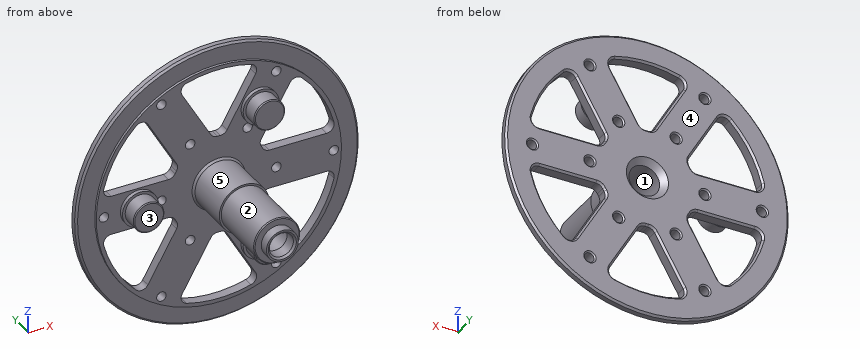
from build123d import *

# Parameters (mm, degrees)
CHAMFER1_SIZE                   = 0.5
CHAMFER2_SIZE                   = 0.25
CIRPATTERN1_COUNT               = 3
CHAMFER2_OF_CIRPATTERN1_SIZE    = 0.25
CHAMFER3_SIZE                   = 0.25
CHAMFER4_SIZE                   = 0.5
M3X0_5_TAPPED_HOLE1_D           = 2.5
M3X0_5_TAPPED_HOLE1_CSINK_D     = 3.2
M3X0_5_TAPPED_HOLE1_CSINK_ANGLE = 90
M3X0_5_TAPPED_HOLE2_D           = 2.5
M3X0_5_TAPPED_HOLE2_CSINK_D     = 3.2
M3X0_5_TAPPED_HOLE2_CSINK_ANGLE = 90
CIRPATTERN2_COUNT               = 6
CUT_EXTRUDE1_DEPTH              = 57.419943282
FILLET1_R                       = 2
CHAMFER5_SIZE                   = 0.5
CIRPATTERN3_COUNT               = 6
FILLET1_OF_CIRPATTERN3_R        = 2
CHAMFER5_OF_CIRPATTERN3_SIZE    = 0.5


with BuildPart() as part:
    # Sketch1 → Revolve1 (revolve)
    with BuildSketch(Plane.XY, mode=Mode.PRIVATE) as revolve1_sk:
        Polygon((-3.15, -8.7), (-4, -8.7), (-4, 19.6), (-5.5, 21.1), (-37, 21.1), (-37, 18.8), (-32, 18.8), (-32, 18.1), (-6.5, 18.1), (-6.5, 6), (-6, 6), (-6, 5.15), (-6, -6), (-6, -7.1), (-6, -9.7), (-4.15, -9.7), (-4.15, -12.2), (-3.15, -12.2), align=None)
    revolve(revolve1_sk.sketch.rotate(Axis((0, 0, 0), (0, -1, 0)), 270), axis=Axis((0, 0, 0), (0, -1, 0)))

    # Chamfer1
    chamfer1_edges = [part.edges().sort_by_distance(p)[0] for p in [
        (0, -12.2, -3.15),
    ]]
    chamfer(chamfer1_edges, length=CHAMFER1_SIZE)

    # Sketch2 → Planet bearing axis (revolve)
    with BuildSketch(Plane.XY):
        Polygon((-21, 18.1), (-25.7, 18.1), (-25.7, 17.1), (-25, 17.1), (-25, 13), (-21, 13), align=None)
    planet_bearing_axis = revolve(axis=Axis((-21, 33.164090746, 0), (0, -1, 0)))

    # Chamfer2
    chamfer2_edges = [part.edges().sort_by_distance(p)[0] for p in [
        (-17, 13, 0),
    ]]
    chamfer(chamfer2_edges, length=CHAMFER2_SIZE)

    # CirPattern1: Planet bearing axis ×3 about axis
    cirpattern1_axis = Axis((0, 0, 0), (0, 1, 0))
    for i in range(1, CIRPATTERN1_COUNT):
        add(planet_bearing_axis.rotate(cirpattern1_axis, i * 360 / CIRPATTERN1_COUNT))

    # Chamfer2 of CirPattern1
    chamfer2_of_cirpattern1_edges = [part.edges().sort_by_distance(p)[0] for p in [
        (8.5, 13, 14.722431864),
        (8.5, 13, -14.722431864),
    ]]
    chamfer(chamfer2_of_cirpattern1_edges, length=CHAMFER2_OF_CIRPATTERN1_SIZE)

    # Chamfer3
    chamfer3_edges = [part.edges().sort_by_distance(p)[0] for p in [
        (0, -9.7, -6),
    ]]
    chamfer(chamfer3_edges, length=CHAMFER3_SIZE)

    # Chamfer4
    chamfer4_edges = [part.edges().sort_by_distance(p)[0] for p in [
        (0, 18.1, -6.5),
        (0, 18.8, -37),
        (0, 21.1, -37),
    ]]
    chamfer(chamfer4_edges, length=CHAMFER4_SIZE)

    # M3x0.5 Tapped Hole1 (through all)
    with Locations(Plane(origin=(0, 21.1, 0), x_dir=(1, 0, 0), z_dir=(0, 1, 0))):
        with Locations((-30, 0)):
            m3x0_5_tapped_hole1 = CounterSinkHole(M3X0_5_TAPPED_HOLE1_D / 2, M3X0_5_TAPPED_HOLE1_CSINK_D / 2, counter_sink_angle=M3X0_5_TAPPED_HOLE1_CSINK_ANGLE)

    # M3x0.5 Tapped Hole2 (through all)
    with Locations(Plane(origin=(0, 21.1, 0), x_dir=(1, 0, 0), z_dir=(0, 1, 0))):
        with Locations((-15, 0)):
            m3x0_5_tapped_hole2 = CounterSinkHole(M3X0_5_TAPPED_HOLE2_D / 2, M3X0_5_TAPPED_HOLE2_CSINK_D / 2, counter_sink_angle=M3X0_5_TAPPED_HOLE2_CSINK_ANGLE)

    # CirPattern2: M3x0.5 Tapped Hole1, M3x0.5 Tapped Hole2 ×6 about axis
    cirpattern2_axis = Axis((0, 0, 0), (0, 1, 0))
    add([m3x0_5_tapped_hole1.rotate(cirpattern2_axis, i * 360 / CIRPATTERN2_COUNT) for i in range(1, CIRPATTERN2_COUNT)], mode=Mode.SUBTRACT)
    add([m3x0_5_tapped_hole2.rotate(cirpattern2_axis, i * 360 / CIRPATTERN2_COUNT) for i in range(1, CIRPATTERN2_COUNT)], mode=Mode.SUBTRACT)

    # Sketch7 → Cut-Extrude1 (cut, through all)
    with BuildSketch(Plane(origin=(0, 0, 0), x_dir=(1, 0, 0), z_dir=(0, 1, 0))):
        with BuildLine():
            Line((-19.745135369, -23.898318544), (-10.428637185, -7.76167034))
            ThreePointArc((-10.428637185, -7.76167034), (-11.258330249, -6.5), (-11.936122283, -5.150629559))
            Line((-11.936122283, -5.150629559), (-30.569118652, -5.150629559))
            ThreePointArc((-30.569118652, -5.150629559), (-26.846787517, -15.5), (-19.745135369, -23.898318544))
        make_face()
    cut_extrude1 = extrude(amount=CUT_EXTRUDE1_DEPTH, mode=Mode.SUBTRACT)

    # Fillet1
    fillet1_edges = [part.edges().sort_by_distance(p)[0] for p in [
        (-30.569118652, 19.6, 5.150629559),
        (-19.745135369, 19.6, 23.898318544),
        (-10.428637185, 19.6, 7.76167034),
        (-11.936122283, 19.6, 5.150629559),
    ]]
    fillet(fillet1_edges, radius=FILLET1_R)

    # Chamfer5
    chamfer5_edges = [part.edges().sort_by_distance(p)[0] for p in [
        (-26.846787517, 21.1, 15.5),
        (-14.783205948, 21.1, 15.304004683),
        (-20.645259809, 21.1, 5.150629559),
        (-11.258330249, 21.1, 6.5),
        (-19.971331194, 21.1, 22.745180132),
        (-29.683569404, 21.1, 5.923090095),
        (-10.785765167, 21.1, 7.817335996),
        (-12.162894146, 21.1, 5.432078636),
    ]]
    chamfer(chamfer5_edges, length=CHAMFER5_SIZE)

    # CirPattern3: Cut-Extrude1 ×6 about axis
    cirpattern3_axis = Axis((0, 0, 0), (0, 1, 0))
    for i in range(1, CIRPATTERN3_COUNT):
        add(cut_extrude1.rotate(cirpattern3_axis, i * 360 / CIRPATTERN3_COUNT), mode=Mode.SUBTRACT)

    # Fillet1 of CirPattern3
    fillet1_of_cirpattern3_edges = [part.edges().sort_by_distance(p)[0] for p in [
        (-10.823983283, 19.6, 29.048948103),
        (10.823983283, 19.6, 29.048948103),
        (1.507485098, 19.6, 12.912299899),
        (-1.507485098, 19.6, 12.912299899),
        (19.745135369, 19.6, 23.898318544),
        (30.569118652, 19.6, 5.150629559),
        (11.936122283, 19.6, 5.150629559),
        (10.428637185, 19.6, 7.76167034),
        (30.569118652, 19.6, -5.150629559),
        (19.745135369, 19.6, -23.898318544),
        (10.428637185, 19.6, -7.76167034),
        (11.936122283, 19.6, -5.150629559),
        (10.823983283, 19.6, -29.048948103),
        (-10.823983283, 19.6, -29.048948103),
        (-1.507485098, 19.6, -12.912299899),
        (1.507485098, 19.6, -12.912299899),
        (-19.745135369, 19.6, -23.898318544),
        (-30.569118652, 19.6, -5.150629559),
        (-11.936122283, 19.6, -5.150629559),
        (-10.428637185, 19.6, -7.76167034),
    ]]
    fillet(fillet1_of_cirpattern3_edges, radius=FILLET1_OF_CIRPATTERN3_R)

    # Chamfer5 of CirPattern3
    chamfer5_of_cirpattern3_edges = [part.edges().sort_by_distance(p)[0] for p in [
        (0, 21.1, 31),
        (5.862053861, 21.1, 20.454634241),
        (-5.862053861, 21.1, 20.454634241),
        (0, 21.1, 13),
        (9.712238211, 21.1, 28.668270227),
        (-9.712238211, 21.1, 28.668270227),
        (1.377128979, 21.1, 13.249414632),
        (-1.377128979, 21.1, 13.249414632),
        (26.846787517, 21.1, 15.5),
        (20.645259809, 21.1, 5.150629559),
        (14.783205948, 21.1, 15.304004683),
        (11.258330249, 21.1, 6.5),
        (29.683569404, 21.1, 5.923090095),
        (19.971331194, 21.1, 22.745180132),
        (12.162894146, 21.1, 5.432078636),
        (10.785765167, 21.1, 7.817335996),
        (26.846787517, 21.1, -15.5),
        (14.783205948, 21.1, -15.304004683),
        (20.645259809, 21.1, -5.150629559),
        (11.258330249, 21.1, -6.5),
        (19.971331194, 21.1, -22.745180132),
        (29.683569404, 21.1, -5.923090095),
        (10.785765167, 21.1, -7.817335996),
        (12.162894146, 21.1, -5.432078636),
        (0, 21.1, -31),
        (-5.862053861, 21.1, -20.454634241),
        (5.862053861, 21.1, -20.454634241),
        (0, 21.1, -13),
        (-9.712238211, 21.1, -28.668270227),
        (9.712238211, 21.1, -28.668270227),
        (-1.377128979, 21.1, -13.249414632),
        (1.377128979, 21.1, -13.249414632),
        (-26.846787517, 21.1, -15.5),
        (-20.645259809, 21.1, -5.150629559),
        (-14.783205948, 21.1, -15.304004683),
        (-11.258330249, 21.1, -6.5),
        (-29.683569404, 21.1, -5.923090095),
        (-19.971331194, 21.1, -22.745180132),
        (-12.162894146, 21.1, -5.432078636),
        (-10.785765167, 21.1, -7.817335996),
    ]]
    chamfer(chamfer5_of_cirpattern3_edges, length=CHAMFER5_OF_CIRPATTERN3_SIZE)


solid = part.part
Source: CAD feature listing. Evaluate the final solid. Frame: model axes, mm. Face numbers are marked on the shaded views. A direction names the side the tool comes from. Round coordinates to 2 decimals unless told otherwise and drop trailing zeros. Loops run counter-clockwise (first coordinate to the right, second up) from the corner with the lowest first, then second, coordinate; pieces in that order, holes last. Notation, with made-up numbers: (86.25, 41.5) - (111.25, 41.5) arc R19 cw to (111.25, 78.5) - close; hole circle Ø5 at (-11, -32.5). An arc over 180 degrees is marked (long way). Write item = value, one per line. Start each with the question number.
(1) Set-up query: the marked faces 4 and 5. Return all of +Z, -Z, +X, -X, +Y, -Y with unobstructed straight access to the full face (end or side cutting, diameter ignored); none if empty.
(2) Pull-direction query (Z, two-part tool) for the marked faces 1, 2 and 3; classes: +Z half, -Z half, draft (parallel to the pull), parting line (faces both ways), or undercut.
(3) Ray query, line 1 along X through (y, z) = (12.5, 0); line 2 along Z through (x, y) = (-7.5, 19.3); line 3 along Y through (x, z) = (-3, -2.5). Return the intervals inside material, ascending. Write a range as from..to.
(4) Section query B-B, the plane z = 19.5. State how many separate pieces and enclosed holes the cut face has, plus the area to 3 significant figures.
(5) Section query A-A, the plane y = 12. Output: boundary loops of the cut face in (x, z).
(6) Pin query (flat end, axial travel): pin 1 (3 mm diameter, centred on x = 22, y = 19, fed in from +Z); pin 2 (3 mm diameter, centred on x = 22.5, z = -25.5, fed in from -Y); pin 3 (3 mm diameter, centred on x = -19.5, y = 19, fed in from +Z). Return the tip coordinate at first contact, or that it passes through.
Conclusion:
q1.face_4 = +Z, -Z, +X, -X, +Y
q1.face_5 = -Y
q2.face_1 = undercut
q2.face_2 = parting line
q2.face_3 = draft
q3.line_1 = -6.5..-4, 4..6.5
q3.line_2 = -36.23..-30.08, -23.29..-14.24, -11.74..11.74, 14.24..23.29, 30.08..36.23
q3.line_3 = -12.2..-8.7
q4.separate_pieces = 4
q4.enclosed_holes = 0
q4.area = 145 mm2
q5.outline = circle Ø13 at (0, 0); hole circle Ø8 at (0, 0)
q6.pin_1 = 30.78
q6.pin_2 = 18.8
q6.pin_3 = 32.31
